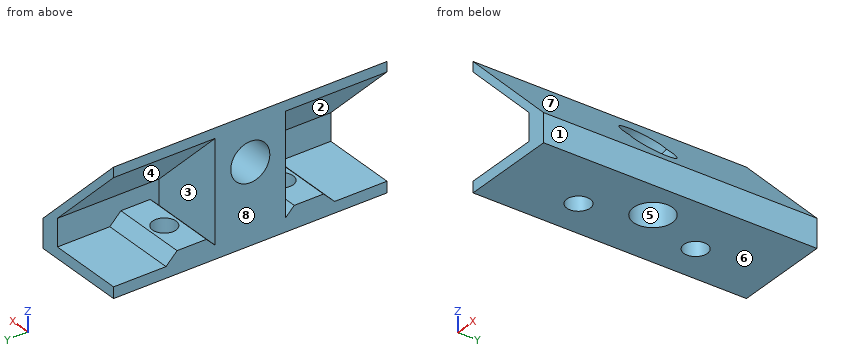
Autodesk Inventor part; units mm, degrees
ref_plane "YZ Plane" through (0, 0, 0) normal (1, 0, 0) x (0, 1, 0)
ref_plane "XZ Plane" through (0, 0, 0) normal (0, 1, 0) x (-1, 0, 0)
ref_plane "XY Plane" through (0, 0, 0) normal (0, 0, 1) x (1, 0, 0)
sketch "Sketch9" plane through (0, 0, 0) normal (0, 1, 0) x (-1, 0, 0)
  line L0 (3.4, -4.445) -> (-1.5, -4.445)
  line L1 (-0.3017, -1.7866) -> (-1.0442, -1.0442) construction
  line L2 (-1.0442, -1.0442) -> (1.7843, 1.7843) construction
  line L3 (1.7843, 1.7843) -> (2.5267, 1.0418) construction
  line L4 (0, 0) -> (0, 4.9841) construction
  line L5 (0, 0) -> (-5.2239, 0) construction
  line L6 (0, 0) -> (1.0887, -0.3962) construction
  line L7 (1.0887, -0.3962) -> (3.6157, -0.3962) construction
  line L8 (-0.3017, -1.7866) -> (2.5267, 1.0418) construction
  line L9 (3.4, 1.9151) -> (-1.5, -2.9849)
  line L10 (-1.5, -2.9849) -> (-1.5, -4.445)
  line L11 (-0.5, -2.494) -> (-0.5, -3.8793)
  line L12 (-0.5, -3.8793) -> (3.4, -3.8793)
  line L13 (3.4, -3.8793) -> (3.4, -4.445)
  line L14 (3.4, -3.8793) -> (2.8343, -4.445) construction
  line L15 (3.4, 1.9151) -> (3.4, 1.406)
  line L16 (3.4, 1.406) -> (-0.5, -2.494)
  line L17 (0, 0) -> (0.5624, -0.5624) construction
  line L18 (3.4, 1.406) -> (3.4, 0.7133)
  line L19 (3.4, 0.7133) -> (-0.5, -3.1867)
  line L20 (3.4, 0.7133) -> (3.4, -3.8793)
  line L21 (0, 0) -> (0.3962, -1.0887) construction
  dimension "d82" = 1.05
  dimension "d83" = 4.445
  dimension "d84" = 3.4
  dimension "d86" = 4
  dimension "d102" = 135
  dimension "d104" = 1
  dimension "d115" = 45
  dimension "d116" = 0.8
  dimension "d125" = 1.5
  dimension "d126" = 0.36
  dimension "d127" = 25
  dimension "d133" = 25
sketch "Sketch14" plane through (0, 0, 0) normal (0, 1, 0) x (-1, 0, 0)
  line L0 (0, 0) -> (0.3962, -1.0887) construction
  line L1 (0, 0) -> (1.0887, -0.3962) construction
  line L2 (0.3962, 3.3492) -> (1.3962, 3.3492)
  line L3 (1.3962, 3.3492) -> (1.3962, -4.9901)
  line L4 (1.3962, -4.9901) -> (0.3962, -4.9901)
  line L5 (0.3962, -4.9901) -> (0.3962, 3.3492)
  line L6 (-1.8344, -0.3962) -> (3.8418, -0.3962)
  line L7 (3.8418, -0.3962) -> (3.8418, -1.3962)
  line L8 (3.8418, -1.3962) -> (-1.8344, -1.3962)
  line L9 (-1.8344, -1.3962) -> (-1.8344, -0.3962)
  dimension "d134" = 1
extrude "Extrusion14" add sketch "Sketch9" along normal mid plane 14 contours L0 L10 L9 L15 L16 L11 L12 L13
sketch "Sketch13" plane through (-3.4, -7, -3.8793) normal (-1, 0, 0) x (0, 0, 1)
  line L0 (0, 0) -> (0, 14)
  line L1 (0, 8.6843) -> (0, 11.3157)
  line L2 (0, 11.3157) -> (0.5657, 10.75)
  line L3 (0.5657, 10.75) -> (0.5657, 9.25)
  line L4 (0.5657, 9.25) -> (0, 8.6843)
  line L5 (0, 7) -> (-0.5657, 7)
  line L6 (-0.5657, 14) -> (0, 14)
  line L7 (0.5657, 10) -> (0, 10) construction
  line L8 (0, 2.6843) -> (0.5657, 3.25)
  line L9 (0.5657, 3.25) -> (0.5657, 4.75)
  line L10 (0.5657, 4.75) -> (0, 5.3157)
  point P0 (3.8793, 7)
  point P1 (-0.2828, 7)
  dimension "d117" = 45
  dimension "d118" = 3
  dimension "d119" = 1.5
extrude "Extrusion16" add sketch "Sketch13" against normal up to next
sketch "Sketch12" plane through (1.5, 7, -4.445) normal (0, 0, -1) x (-1, 0, 0)
  circle A0 centre (3, -4) radius 0.6
  circle A1 centre (3, -10) radius 0.6
  point P0 (1.5, -7)
  dimension "d109" = 1.5
  dimension "d110" = 3
  dimension "d111" = 3
  dimension "d112" = 1.2
extrude "Extrusion15" cut sketch "Sketch12" against normal blind 2
extrude "Extrusion17" add sketch "Sketch9" along normal mid plane 3.6 contours L12 L11 L19 L20 | L19 L11 L16 L18
revolve "Revolution5" cut sketch "Sketch14" angle 360 about axis through (-0.3962, 0, -4.9901) along (0, 0, 1) contours L2 L3 L6 L5 | L6 L3 L8 L5 | L8 L3 L4 L5
revolve "Revolution6" cut sketch "Sketch14" angle 360 about axis through (1.8344, 0, -0.3962) along (-1, 0, 0) contours L6 L3 L8 L5 | L5 L8 L9 L6 | L6 L7 L8 L3
properties part number "round dichroic holder"
The model under review builds one solid part; all positions refer to its coordinate system, in mm. Face numbers are marked on the shaded views. A direction names the side the tool comes from. Round coordinates to 2 decimals unless told otherwise and drop trailing zeros. Loops run counter-clockwise (first coordinate to the right, second up) from the corner with the lowest first, then second, coordinate; pieces in that order, holes last. Notation, with made-up numbers: (-4.5, 41) -> (25.5, 41) arc R17 ccw to (25.5, 68) -> close; hole circle Ø9 at (-30.5, -2). An arc over 180 degrees is marked (long way). Answer as CSV lines item,"result".
1) Add section A-A on y = 3. Write out the cut boundary in (x, z) (3 decimals).
Geometry results:
outline,"(-3.4, -4.445) -> (-2.1, -4.445) -> (-2.1, -3.314) -> (-3.4, -3.314) -> close; (-3.4, 1.406) -> (0.5, -2.494) -> (0.5, -3.314) -> (-0.9, -3.314) -> (-0.9, -4.445) -> (1.5, -4.445) -> (1.5, -2.985) -> (-3.4, 1.915) -> close"
2) Add section C-C on x = 0.3. Write out the cut boundary in (y, z) (3 decimals).
Geometry results:
outline,"(-7, -4.445) -> (-0.718, -4.445) -> (-0.718, -1.785) -> (-7, -1.785) -> (-7, -2.294) -> (-1.8, -2.294) -> (-1.8, -3.764) -> (-2.25, -3.314) -> (-3.75, -3.314) -> (-4.316, -3.879) -> (-7, -3.879) -> close; (0.718, -4.445) -> (7, -4.445) -> (7, -3.879) -> (4.316, -3.879) -> (3.75, -3.314) -> (2.25, -3.314) -> (1.8, -3.764) -> (1.8, -2.294) -> (7, -2.294) -> (7, -1.785) -> (0.718, -1.785) -> close"
3) Tool access review of the marked faces 1, 2, 3 and 4: name each direction out of +Z, -Z, +X, -X, +Y, -Y from which nothing blocks a thin tool from reaching the whole face with its end or side.
Geometry results:
face 1,"+Z, -Z, +X, +Y, -Y"
face 2,"-X, -Y"
face 3,"-X"
face 4,"-X, +Y"
4) Add section D-D on y = 0. Write out the cut boundary in (x, z) (3 decimals), plus the area to 3 significant figures.
Geometry results:
outline,"(-3.4, -4.445) -> (-1.396, -4.445) -> (-1.396, -1.396) -> (-3.4, -1.396) -> close; (-3.4, 0.604) -> (-2.089, 0.604) -> (-3.4, 1.915) -> close; (0.604, -4.445) -> (1.5, -4.445) -> (1.5, -2.985) -> (0.604, -2.089) -> close"
area,"8.68 mm²"
5) Draft analysis for pull direction X (two halves, no side actions). For the marked faces 5, 6, 7 and 8, state which applies: pulls with the +X half, pulls with the -X half, needs draft (parallel to the pull), parting line crosses it, or undercut.
Geometry results:
face 5,"undercut"
face 6,"needs draft"
face 7,"pulls with the +X half"
face 8,"pulls with the -X half"
6) For P1, Ø1.1, axis at y = 5, z = -3, coming from the -X side; P2, Ø1.5, axis at y = -5, z = -3, coming from the -X side; P3, Ø1.6, axis at x = -2, y = 3, coming from the +Z side, all flat-tipped, find the tip position at first contact; note any pin that passes through.
Geometry results:
P1,"stops at x = 0.46"
P2,"stops at x = 0.26"
P3,"stops at z = 1.32"
7) Add section B-B on z = 0. Write out the cut boundary in (x, y), plus the area to 3 significant figures.
Geometry results:
outline,"(-3.4, -1.8) -> (-1.99, -1.8) -> (-1.99, -7) -> (-1.48, -7) -> (-1.48, -0.92) -> (-3.4, -0.92) -> close; (-3.4, 0.92) -> (-1.48, 0.92) -> (-1.48, 7) -> (-1.99, 7) -> (-1.99, 1.8) -> (-3.4, 1.8) -> close"
area,"8.67 mm²"
8) To check wall thickness, follow line 1 along Y through (x, z) = (-1.5, -4.1); line 2 along X through (y, z) = (0, -3.6); line 3 along Y through (x, z) = (-1.5, -3.6). State the ranges of each line that lie inside material, in increasing order. Write a range as from..to.
Geometry results:
line 1,"y = -7..-3.6, -2.4..2.4, 3.6..7"
line 2,"x = -3.4..-1.4, 0.6..1.5"
line 3,"y = -4.04..-3.6, -2.4..-1.96, -1.8..1.8, 1.96..2.4, 3.6..4.04"
